Build history of the part. All positions in model axes, mm. A direction names the side the tool comes from. Round coordinates to 2 decimals unless told otherwise and drop trailing zeros. Loops run counter-clockwise (first coordinate to the right, second up) from the corner with the lowest first, then second, coordinate; pieces in that order, holes last. Notation, with made-up numbers: (65.5, 26.25) - (72.5, 26.25) arc R23 ccw to (72.5, 57.25) - close; hole circle Ø6 at (-2.5, -34.75). An arc over 180 degrees is marked (long way). Use one line per item in the form item = value. Start each with the question number.
Q1. Saw through at B-B (y = 8.75). Give the cut face in (x, z) (3 decimals).
Q2. Saw through at C-C (z = 0.45). Give the cut face in (x, y).
Q3. 3-axis set-ups, long thin cutter, end or side, ignore diameter. For faces 1 (the face through (12, -2.5, 0)), 2 (the face through (9.3, 4.1, -0.675)), 3 (the face through (12, 0.5, 0)), 4 (the face through (12, 2.5, 0)), 5 (the face through (-11, 0, 0)): which of +Z, -Z, +X, -X, +Y, -Y reach the whole face in a straight line?
Q4. Mould opens along X. For faces 6 (the face through (12, -1, 0)), 7 (the face through (13.33, 1.58, 0.01)), 8 (the face through (9.3, 4.1, 0.675)) say: released by +X, released by -X, zero draft, split by the parting line, or undercut.
Q5. Saw through at D-D (y = 1.5). Give the cut face in (x, z) (1 decimal).
Q6. Drill centre lines: line 1 (Y direction, x = 12, z = -0.35); line 2 (X direction, y = 1.25, z = 0.1); line 3 (X direction, y = 1.5, z = 0.25). Where is each one in solid material? Low to high.
Q7. Saw through at A-A (x = 0). Give the cut face in (y, z) (3 decimals), then the cut area to 3 significant figures.
```python
from build123d import *

# Parameters (mm, degrees)
SKETCH1_R           = 0.5
BOSS_EXTRUDE1_DEPTH = 0.675


with BuildPart() as part:
    # Sketch1 → Boss-Extrude1 (new, symmetric)
    with BuildSketch(Plane(origin=(0, 0, 0), x_dir=(0, 1, 0), z_dir=(0, 0, 1))):
        with BuildLine():
            Line((-0.5, -10.45227248), (-0.5, -12.904865966))
            ThreePointArc((-0.5, -12.904865966), (-0.671970486, -13.282220756), (-1.06958655, -13.4))
            Line((-1.06958655, -13.4), (-2.06958655, -13.259459165))
            ThreePointArc((-2.06958655, -13.259459165), (-2.37735479, -13.092354645), (-2.5, -12.764325131))
            Line((-2.5, -12.764325131), (-2.5, -11.101801656))
            ThreePointArc((-2.5, -11.101801656), (-2.603000383, -10.797842276), (-2.869565217, -10.619114627))
            ThreePointArc((-2.869565217, -10.619114627), (0, 11), (2.869565217, -10.619114627))
            ThreePointArc((2.869565217, -10.619114627), (2.603000383, -10.797842276), (2.5, -11.101801656))
            Line((2.5, -11.101801656), (2.5, -12.764325131))
            ThreePointArc((2.5, -12.764325131), (2.37735479, -13.092354645), (2.06958655, -13.259459165))
            Line((2.06958655, -13.259459165), (1.06958655, -13.4))
            ThreePointArc((1.06958655, -13.4), (0.671970486, -13.282220756), (0.5, -12.904865966))
            Line((0.5, -12.904865966), (0.5, -10.45227248))
            ThreePointArc((0.5, -10.45227248), (0.629993565, -10.115976126), (0.952380952, -9.954545219))
            ThreePointArc((0.952380952, -9.954545219), (0, 10), (-0.952380952, -9.954545219))
            ThreePointArc((-0.952380952, -9.954545219), (-0.629993565, -10.115976126), (-0.5, -10.45227248))
        make_face()
        with Locations(Location((-1.5, -12, 0), (0, 0, 270))):
            Circle(SKETCH1_R, mode=Mode.SUBTRACT)
        with Locations(Location((1.5, -12, 0), (0, 0, 90))):
            Circle(SKETCH1_R, mode=Mode.SUBTRACT)
    extrude(amount=BOSS_EXTRUDE1_DEPTH, both=True)


solid = part.part
```
Report:
q1.outline = (-6.666, -0.675) - (-4.841, -0.675) - (-4.841, 0.675) - (-6.666, 0.675) - close; (4.841, -0.675) - (6.666, -0.675) - (6.666, 0.675) - (4.841, 0.675) - close
q2.outline = (9.95, -0.95) arc R10 cw (long way) to (9.95, 0.95) arc R0.5 ccw to (10.45, 0.5) - (12.9, 0.5) arc R0.5 ccw to (13.4, 1.07) - (13.26, 2.07) arc R0.5 ccw to (12.76, 2.5) - (11.1, 2.5) arc R0.5 cw to (10.62, 2.87) arc R11 ccw (long way) to (10.62, -2.87) arc R0.5 cw to (11.1, -2.5) - (12.76, -2.5) arc R0.5 ccw to (13.26, -2.07) - (13.4, -1.07) arc R0.5 ccw to (12.9, -0.5) - (10.45, -0.5) arc R0.5 ccw to start; hole circle Ø1 at (12, -1.5); hole circle Ø1 at (12, 1.5)
q3.face_1 = +Z, -Z, +X, -Y
q3.face_2 = -Z, +X, -X, +Y, -Y
q3.face_3 = +Z, -Z, +X
q3.face_4 = +Z, -Z, +X, +Y
q3.face_5 = +Z, -Z
q4.face_6 = undercut
q4.face_7 = released by +X
q4.face_8 = zero draft
q5.outline = (-10.9, -0.7) - (-9.9, -0.7) - (-9.9, 0.7) - (-10.9, 0.7) - close; (9.9, -0.7) - (11.5, -0.7) - (11.5, 0.7) - (9.9, 0.7) - close; (12.5, -0.7) - (13.3, -0.7) - (13.3, 0.7) - (12.5, 0.7) - close
q6.line_1 = -2.5 to -2, -1 to -0.5, 0.5 to 1, 2 to 2.5
q6.line_2 = -10.93 to -9.92, 9.92 to 11.57, 12.43 to 13.37
q6.line_3 = -10.9 to -9.89, 9.89 to 11.5, 12.5 to 13.34
q7.outline = (-11, -0.675) - (-10, -0.675) - (-10, 0.675) - (-11, 0.675) - close; (10, -0.675) - (11, -0.675) - (11, 0.675) - (10, 0.675) - close
q7.area = 2.70 mm²
